The model under review builds one solid part; all positions refer to its coordinate system, in mm. A direction names the side the tool comes from. Give positions to 0.01 mm unless a question says otherwise; leave off trailing zeros. Loops run counter-clockwise (first coordinate to the right, second up) from the corner with the lowest first, then second, coordinate; pieces in that order, holes last. Notation, with made-up numbers: (20, 63) -> (65, 63) arc R23 ccw to (65, 93) -> close; hole circle Ø2 at (3, 42.5). An arc over 180 degrees is marked (long way). Write each question's results on one line, items separated by ' | '. Start each with the question number.
Q1. We need section B-B (y = 10.5). Write out the cut boundary in (x, z).
Q2. Machinability: for faces 5 (the face through (-33, 27, -40.018)), 6 (the face through (-65, 34, -17.018)), 7 (the face through (-107.678, 12, -33)), 8 (the face through (-24.8, 28.5, -30.7)), which of the approach directions +Z, -Z, +X, -X, +Y, -Y give a long, thin tool a straight path to every point of the face, cutting with its end or side? Answer none if there is none.
Q3. Wall thickness on L1, parallel to Z at x = -12.5, y = 3; L2, parallel to Y at x = -61, z = -35; L3, parallel to X at y = 5, z = -46: over which ranges is each line inside the solid? List them lowest first. Write a range as [from, to].
Q4. Mouldability with a two-part tool opening along Y and no side actions: class faces 1 (the face through (-75.451, 13.339, -45.483)), 2 (the face through (-102, 38, -15)), 3 (the face through (-108, 25, -48.018)), 4 (the face through (-66.044, 15.737, -15.483)) as released by +Y, released by -Y, zero draft, split by the parting line, or undercut.
Q5. We need section A-A (x = -50.5). Write out the cut boundary in (y, z).
Q6. We need section C-C (z = -30.5). Write out the cut boundary in (x, y), plus the area to 3 significant figures.
Q7. We need section D-D (y = 16.5). Write out the cut boundary in (x, z).
Q8. Insertion check: pin 1 Ø1.3 at (x, y) = (-101, 24) entering from -Z; pin 2 Ø12 at (x, z) = (-32, -16) entering from +Y; pin 3 Ø2 at (y, z) = (26.5, -35) entering from +X; pin 4 Ø1 at (x, z) = (-59.5, -11.5) entering from -Y. Each pin has a flat end and moves straight along its axis. Give the tip position at first contact, or say it passes through.
from build123d import *

# Parameters (mm, degrees)
BOSS_EXTRUDE3_DEPTH       = 30
SKETCH6_W                 = 25
SKETCH6_H                 = 23
CUT_EXTRUDE1_DEPTH        = 86
SKETCH7_W                 = 25
SKETCH7_H                 = 5
CUT_EXTRUDE2_DEPTH        = 7.5
SKETCH8_W                 = 25
SKETCH8_H                 = 2
CUT_EXTRUDE3_DEPTH        = 1
SKETCH9_R                 = 19
CUT_EXTRUDE4_DEPTH        = 5
BOSS_EXTRUDE4_DEPTH       = 30
SKETCH10_W                = 1.856561782
SKETCH10_H                = 30
BOSS_EXTRUDE5_DEPTH       = 3
BOSS_EXTRUDE6_DEPTH       = 30
SKETCH11_W                = 2.5
SKETCH11_H                = 23
CUT_EXTRUDE5_DEPTH        = 34.579503854
SKETCH12_W                = 29.135235428
SKETCH12_H                = 25
CUT_EXTRUDE6_DEPTH        = 3.5
SKETCH13_W                = 19.135235428
SKETCH13_H                = 5
CUT_EXTRUDE7_DEPTH        = 3.5
SKETCH14_W                = 29.135235428
SKETCH14_H                = 4
BOSS_EXTRUDE7_DEPTH       = 2
SKETCH16_W                = 29.135235428
SKETCH16_H                = 1.5
BOSS_EXTRUDE8_DEPTH       = 2
SKETCH17_W                = 2.551467674
SKETCH17_H                = 30
BOSS_EXTRUDE9_DEPTH       = 5
BOSS_EXTRUDE10_REACH      = 85.266
SKETCH18_W                = 29.135235428
SKETCH18_H                = 2.5
SKETCH19_W                = 2.48850009
SKETCH19_H                = 23
BOSS_EXTRUDE11_DEPTH      = 2
CUT_EXTRUDE8_START        = -2.4885
SKETCH20_W                = 2
SKETCH20_H                = 23
CUT_EXTRUDE8_DEPTH        = 21.736568
BOSS_EXTRUDE12_REACH      = 82.714
SKETCH21_W                = 2.023287715
SKETCH21_H                = 27.5
SKETCH22_W                = 35
SKETCH22_H                = 30
BOSS_EXTRUDE13_DEPTH      = 15.9
BOSS_EXTRUDE13_DEPTH_BACK = 7.5
SKETCH23_W                = 25
SKETCH23_H                = 23
CUT_EXTRUDE9_DEPTH        = 24.4
SKETCH24_W                = 25
SKETCH24_H                = 5
CUT_EXTRUDE10_DEPTH       = 2
SKETCH25_W                = 50
SKETCH25_H                = 29
CUT_EXTRUDE11_DEPTH       = 4
SKETCH26_W                = 3
SKETCH26_H                = 29
BOSS_EXTRUDE14_DEPTH      = 2.5
SKETCH27_W                = 5
SKETCH27_H                = 5
BOSS_EXTRUDE15_DEPTH      = 2.5
BOSS_EXTRUDE16_REACH      = 27
SKETCH28_W                = 4
SKETCH28_H                = 2.5
SKETCH29_W                = 13
SKETCH29_H                = 5
BOSS_EXTRUDE17_DEPTH      = 2.5
SKETCH30_W                = 10
SKETCH30_H                = 4
CUT_EXTRUDE12_DEPTH       = 14
CUT_EXTRUDE13_REACH       = 43.166
SKETCH31_W                = 10
SKETCH31_H                = 2
SKETCH32_W                = 2
SKETCH32_H                = 25
CUT_EXTRUDE14_DEPTH       = 27
SKETCH33_W                = 20.479278159
SKETCH33_H                = 4
BOSS_EXTRUDE18_DEPTH      = 8
SKETCH34_W                = 15.845031547
SKETCH34_H                = 4
BOSS_EXTRUDE19_DEPTH      = 8


with BuildPart() as part:
    # Sketch2 → Boss-Extrude3 (new body)
    with BuildSketch(Plane(origin=(0, 0, 0), x_dir=(1, 0, 0), z_dir=(0, 1, 0))):
        Polygon((-105.912162162, 13.018018018), (-20.912162162, 13.018018018), (-20.912162162, 48.018018018), (-75.912162162, 48.018018018), align=None)
    extrude(amount=BOSS_EXTRUDE3_DEPTH)

    # Sketch6 → Cut-Extrude1 (cut, through all)
    with BuildSketch(Plane(origin=(-20.912162162, 0, 0), x_dir=(0, 0, -1), z_dir=(1, 0, 0))):
        with Locations((30.518018018, 13.5)):
            Rectangle(SKETCH6_W, SKETCH6_H)
    extrude(amount=-CUT_EXTRUDE1_DEPTH, mode=Mode.SUBTRACT)

    # Sketch7 → Cut-Extrude2 (cut)
    with BuildSketch(Plane(origin=(-20.912162162, 0, 0), x_dir=(0, 0, -1), z_dir=(1, 0, 0))):
        with Locations((30.518018018, 27.5)):
            Rectangle(SKETCH7_W, SKETCH7_H)
    extrude(amount=-CUT_EXTRUDE2_DEPTH, mode=Mode.SUBTRACT)

    # Sketch8 → Cut-Extrude3 (cut)
    with BuildSketch(Plane(origin=(-20.912162162, 0, 0), x_dir=(0, 0, -1), z_dir=(1, 0, 0))):
        with Locations((30.518018018, 1)):
            Rectangle(SKETCH8_W, SKETCH8_H)
    extrude(amount=-CUT_EXTRUDE3_DEPTH, mode=Mode.SUBTRACT)

    # Sketch9 → Cut-Extrude4 (cut)
    with BuildSketch(Plane.XY.offset(-13.018018018)):
        with Locations((-84.912162162, 13.5)):
            Circle(SKETCH9_R)
    extrude(amount=-CUT_EXTRUDE4_DEPTH, mode=Mode.SUBTRACT)

    # Sketch3 → Boss-Extrude4 (add)
    with BuildSketch(Plane(origin=(0, 0, 0), x_dir=(1, 0, 0), z_dir=(0, 1, 0))):
        Polygon((-106.412808957, 7.383361614), (-110.17791555, 11.88278259), (-79.204856611, 48.018018018), (-75.912162162, 48.018018018), (-105.912162162, 13.018018018), (-103.345157358, 9.950366419), align=None)
    extrude(amount=BOSS_EXTRUDE4_DEPTH)

    # Sketch10 → Boss-Extrude5 (add)
    with BuildSketch(Plane.XY.offset(-13.018018018)):
        with Locations((-104.983881271, 15)):
            Rectangle(SKETCH10_W, SKETCH10_H)
    extrude(amount=BOSS_EXTRUDE5_DEPTH)

    # Sketch4 → Boss-Extrude6 (add)
    with BuildSketch(Plane(origin=(0, 0, 0), x_dir=(1, 0, 0), z_dir=(0, 1, 0))):
        Polygon((-110.17791555, 11.88278259), (-110.17791555, 48.018018018), (-104.17791555, 48.018018018), (-104.17791555, 18.88278259), align=None)
    extrude(amount=BOSS_EXTRUDE6_DEPTH)

    # Sketch11 → Cut-Extrude5 (cut, through all)
    with BuildSketch(Plane(origin=(-47.459390138, 0, -56.715466139), x_dir=(0.7669129, 0, -0.641751201), z_dir=(0.641751201, 0, 0.7669129))):
        with Locations((-74.121074711, 13.5)):
            Rectangle(SKETCH11_W, SKETCH11_H)
    extrude(amount=-CUT_EXTRUDE5_DEPTH, mode=Mode.SUBTRACT)

    # Sketch12 → Cut-Extrude6 (cut)
    with BuildSketch(Plane(origin=(-104.17791555, 0, 0), x_dir=(0, 0, -1), z_dir=(1, 0, 0))):
        with Locations((33.450400304, 15)):
            Rectangle(SKETCH12_W, SKETCH12_H)
    extrude(amount=-CUT_EXTRUDE6_DEPTH, mode=Mode.SUBTRACT)

    # Sketch13 → Cut-Extrude7 (cut, through all)
    with BuildSketch(Plane(origin=(-107.67791555, 0, 0), x_dir=(0, 0, -1), z_dir=(1, 0, 0))):
        with Locations((38.450400304, 15)):
            Rectangle(SKETCH13_W, SKETCH13_H)
    extrude(amount=-CUT_EXTRUDE7_DEPTH, mode=Mode.SUBTRACT)

    # Sketch14 → Boss-Extrude7 (add)
    with BuildSketch(Plane(origin=(-107.67791555, 0, 0), x_dir=(0, 0, -1), z_dir=(1, 0, 0))):
        with Locations((33.450400304, 25.5)):
            Rectangle(SKETCH14_W, SKETCH14_H)
    extrude(amount=BOSS_EXTRUDE7_DEPTH)

    # Sketch16 → Boss-Extrude8 (add)
    with BuildSketch(Plane(origin=(-107.67791555, 0, 0), x_dir=(0, 0, -1), z_dir=(1, 0, 0))):
        with Locations((33.450400304, 3.25)):
            Rectangle(SKETCH16_W, SKETCH16_H)
    extrude(amount=BOSS_EXTRUDE8_DEPTH)

    # Sketch17 → Boss-Extrude9 (add)
    with BuildSketch(Plane(origin=(0, 0, -18.88278259), x_dir=(-1, 0, 0), z_dir=(0, 0, -1))):
        with Locations((102.902181713, 15)):
            Rectangle(SKETCH17_W, SKETCH17_H)
    extrude(amount=BOSS_EXTRUDE9_DEPTH)

    # Boss-Extrude10: up to this face of the body (flat: up to its plane)
    boss_extrude10_end = Plane(part.part.faces().sort_by_distance((-90.415652244, 15, -34.938756447))[0])
    # Sketch18 → Boss-Extrude10 (add, up to the picked face)
    with BuildSketch(Plane(origin=(-104.17791555, 0, 0), x_dir=(0, 0, -1), z_dir=(1, 0, 0)), mode=Mode.PRIVATE) as boss_extrude10_sk1:
        with Locations((33.450400304, 1.25)):
            Rectangle(SKETCH18_W, SKETCH18_H)
    boss_extrude10_tool1 = split(extrude(boss_extrude10_sk1.sketch, amount=BOSS_EXTRUDE10_REACH, mode=Mode.PRIVATE), bisect_by=boss_extrude10_end, keep=Keep.BOTH, mode=Mode.PRIVATE)
    add(boss_extrude10_tool1.solids().sort_by_distance((-104.177916, 1.25, -33.4504))[0])

    # Sketch19 → Boss-Extrude11 (add)
    with BuildSketch(Plane(origin=(-67.487678855, 0, -57.846581876), x_dir=(0.650791373, 0, -0.759256602), z_dir=(0.759256602, 0, 0.650791373))):
        with Locations((-31.723015124, 13.5)):
            Rectangle(SKETCH19_W, SKETCH19_H)
    extrude(amount=BOSS_EXTRUDE11_DEPTH)

    # Sketch20 → Cut-Extrude8 (cut)
    with BuildSketch(Plane(origin=(-19.835317387, 0, 23.141203618), x_dir=(-0.759256602, 0, -0.650791373), z_dir=(0.650791373, 0, -0.759256602)).offset(CUT_EXTRUDE8_START)):
        with Locations((87.886522218, 13.5)):
            Rectangle(SKETCH20_W, SKETCH20_H)
    extrude(amount=CUT_EXTRUDE8_DEPTH, mode=Mode.SUBTRACT)

    # Boss-Extrude12: up to this face of the body (flat: up to its plane)
    boss_extrude12_end = Plane(part.part.faces().sort_by_distance((-90.415652244, 16.25, -34.938756447))[0])
    # Sketch21 → Boss-Extrude12 (add, up to the picked face)
    with BuildSketch(Plane(origin=(-101.626447876, 0, 0), x_dir=(0, 0, -1), z_dir=(1, 0, 0)), mode=Mode.PRIVATE) as boss_extrude12_sk1:
        with Locations((22.871138733, 16.25)):
            Rectangle(SKETCH21_W, SKETCH21_H)
    boss_extrude12_tool1 = split(extrude(boss_extrude12_sk1.sketch, amount=BOSS_EXTRUDE12_REACH, mode=Mode.PRIVATE), bisect_by=boss_extrude12_end, keep=Keep.BOTH, mode=Mode.PRIVATE)
    add(boss_extrude12_tool1.solids().sort_by_distance((-101.626448, 16.25, -22.871139))[0])

    # Sketch22 → Boss-Extrude13 (add, two sides)
    with BuildSketch(Plane(origin=(-20.912162162, 0, 0), x_dir=(0, 0, -1), z_dir=(1, 0, 0))) as boss_extrude13_sk:
        with Locations((30.518018018, 15)):
            Rectangle(SKETCH22_W, SKETCH22_H)
    extrude(amount=BOSS_EXTRUDE13_DEPTH)
    extrude(boss_extrude13_sk.sketch, amount=-BOSS_EXTRUDE13_DEPTH_BACK)

    # Sketch23 → Cut-Extrude9 (cut, through all)
    with BuildSketch(Plane.ZY.offset(28.412162162)):
        with Locations((-30.518018018, 13.5)):
            Rectangle(SKETCH23_W, SKETCH23_H)
    extrude(amount=-CUT_EXTRUDE9_DEPTH, mode=Mode.SUBTRACT)

    # Sketch24 → Cut-Extrude10 (cut)
    with BuildSketch(Plane(origin=(-5.012162162, 0, 0), x_dir=(0, 0, -1), z_dir=(1, 0, 0))):
        with Locations((30.518018018, 27.5)):
            Rectangle(SKETCH24_W, SKETCH24_H)
    extrude(amount=-CUT_EXTRUDE10_DEPTH, mode=Mode.SUBTRACT)

    # Sketch25 → Cut-Extrude11 (cut)
    with BuildSketch(Plane(origin=(0, 30, 0), x_dir=(1, 0, 0), z_dir=(0, 1, 0))):
        with Locations((-30.012162162, 30.518018018)):
            Rectangle(SKETCH25_W, SKETCH25_H)
    extrude(amount=-CUT_EXTRUDE11_DEPTH, mode=Mode.SUBTRACT)

    # Sketch26 → Boss-Extrude14 (add)
    with BuildSketch(Plane(origin=(0, 26, 0), x_dir=(1, 0, 0), z_dir=(0, 1, 0))):
        with Locations((-23.512162162, 30.518018018)):
            Rectangle(SKETCH26_W, SKETCH26_H)
    extrude(amount=BOSS_EXTRUDE14_DEPTH)

    # Sketch27 → Boss-Extrude15 (add)
    with BuildSketch(Plane(origin=(0, 26, 0), x_dir=(1, 0, 0), z_dir=(0, 1, 0))):
        with Locations((-32.512162162, 42.518018018)):
            Rectangle(SKETCH27_W, SKETCH27_H)
    extrude(amount=BOSS_EXTRUDE15_DEPTH)

    # Sketch28 → Boss-Extrude16 (add, up to next)
    with BuildSketch(Plane(origin=(-30.012162162, 0, 0), x_dir=(0, 0, -1), z_dir=(1, 0, 0)), mode=Mode.PRIVATE) as boss_extrude16_sk1:
        with Locations((43.018018018, 27.25)):
            Rectangle(SKETCH28_W, SKETCH28_H)
    boss_extrude16_tool1 = extrude(boss_extrude16_sk1.sketch, amount=BOSS_EXTRUDE16_REACH, mode=Mode.PRIVATE) - part.part
    add(boss_extrude16_tool1.solids().sort_by_distance((-30.012162, 27.25, -43.018018))[0])

    # Sketch29 → Boss-Extrude17 (add)
    with BuildSketch(Plane(origin=(0, 26, 0), x_dir=(1, 0, 0), z_dir=(0, 1, 0))):
        with Locations((-31.512162162, 18.518018018)):
            Rectangle(SKETCH29_W, SKETCH29_H)
    extrude(amount=BOSS_EXTRUDE17_DEPTH)

    # Sketch30 → Cut-Extrude12 (cut)
    with BuildSketch(Plane(origin=(-55.012162162, 0, 0), x_dir=(0, 0, -1), z_dir=(1, 0, 0))):
        with Locations((37.018018018, 28)):
            Rectangle(SKETCH30_W, SKETCH30_H)
    extrude(amount=-CUT_EXTRUDE12_DEPTH, mode=Mode.SUBTRACT)

    # Sketch31 → Cut-Extrude13 (cut, up to next)
    with BuildSketch(Plane(origin=(-69.012162162, 0, 0), x_dir=(0, 0, -1), z_dir=(1, 0, 0)), mode=Mode.PRIVATE) as cut_extrude13_sk1:
        with Locations((37.018018018, 29)):
            Rectangle(SKETCH31_W, SKETCH31_H)
    cut_extrude13_tool1 = extrude(cut_extrude13_sk1.sketch, amount=-CUT_EXTRUDE13_REACH, mode=Mode.PRIVATE) & part.part
    add(cut_extrude13_tool1.solids().sort_by_distance((-69.012162, 29, -37.018018))[0], mode=Mode.SUBTRACT)

    # Sketch32 → Cut-Extrude14 (cut, through all)
    with BuildSketch(Plane(origin=(0, 26, 0), x_dir=(1, 0, 0), z_dir=(0, 1, 0))):
        with Locations((-6.012162162, 30.518018018)):
            Rectangle(SKETCH32_W, SKETCH32_H)
    extrude(amount=-CUT_EXTRUDE14_DEPTH, mode=Mode.SUBTRACT)

    # Sketch33 → Boss-Extrude18 (add)
    with BuildSketch(Plane(origin=(0, 30, 0), x_dir=(1, 0, 0), z_dir=(0, 1, 0))):
        with Locations((-65.251801242, 15.018018018)):
            Rectangle(SKETCH33_W, SKETCH33_H)
    extrude(amount=BOSS_EXTRUDE18_DEPTH)

    # Sketch34 → Boss-Extrude19 (add)
    with BuildSketch(Plane(origin=(0, 30, 0), x_dir=(1, 0, 0), z_dir=(0, 1, 0))):
        with Locations((-102.255399777, 15.018018018)):
            Rectangle(SKETCH34_W, SKETCH34_H)
    extrude(amount=BOSS_EXTRUDE19_DEPTH)


solid = part.part
Output:
1) outline: (-110.18, -48.02) -> (-107.68, -48.02) -> (-107.68, -18.88) -> (-104.18, -18.88) -> (-104.18, -23.88) -> (-99.89, -23.88) -> (-79.2, -48.02) -> (-75.91, -48.02) -> (-103.67, -15.63) -> (-103.67, -13.02) -> (-104.06, -13.02) -> (-104.06, -10.8) -> (-110.18, -18.12) -> close; (-110.18, -14.22) -> (-105.26, -8.35) -> (-106.41, -7.38) -> (-110.18, -11.88) -> close; (-77.56, -43.02) -> (-73.28, -48.02) -> (-5.01, -48.02) -> (-5.01, -43.02) -> close; (-66.15, -18.02) -> (-5.01, -18.02) -> (-5.01, -13.02) -> (-66.15, -13.02) -> close
2) face 5: +Y | face 6: -Z, +X, -X, +Y | face 7: -Z | face 8: +X, +Y
3) L1: [-48.02, -43.02], [-18.02, -13.02] | L2: [0, 2], [25, 26] | L3: [-110.18, -107.68], [-80.93, -77.64], [-75.01, -5.01]
4) face 1: undercut | face 2: released by +Y | face 3: zero draft | face 4: undercut
5) outline: (0, -48.02) -> (30, -48.02) -> (30, -45.02) -> (26, -45.02) -> (26, -16.02) -> (30, -16.02) -> (30, -13.02) -> (0, -13.02) -> close; hole (2, -43.02) -> (25, -43.02) -> (25, -18.02) -> (2, -18.02) -> close
6) outline: (-110.18, 0) -> (-7.01, 0) -> (-7.01, 2) -> (-90.93, 2) -> (-90.93, 25) -> (-7.01, 25) -> (-7.01, 26) -> (-22.01, 26) -> (-22.01, 28.5) -> (-25.01, 28.5) -> (-25.01, 26) -> (-55.01, 26) -> (-55.01, 30) -> (-94.22, 30) -> (-94.22, 2.5) -> (-105.68, 2.5) -> (-105.68, 4) -> (-107.68, 4) -> (-107.68, 12.5) -> (-110.18, 12.5) -> close; (-110.18, 17.5) -> (-107.68, 17.5) -> (-107.68, 23.5) -> (-105.68, 23.5) -> (-105.68, 27.5) -> (-104.18, 27.5) -> (-104.18, 30) -> (-110.18, 30) -> close | area: 618 mm2
7) outline: (-110.18, -28.88) -> (-107.68, -28.88) -> (-107.68, -18.88) -> (-104.18, -18.88) -> (-104.18, -23.88) -> (-99.89, -23.88) -> (-79.2, -48.02) -> (-75.91, -48.02) -> (-103.67, -15.63) -> (-103.67, -13.02) -> (-104.06, -13.02) -> (-104.06, -10.8) -> (-110.18, -18.12) -> close; (-110.18, -14.22) -> (-105.26, -8.35) -> (-106.41, -7.38) -> (-110.18, -11.88) -> close; (-77.56, -43.02) -> (-73.28, -48.02) -> (-5.01, -48.02) -> (-5.01, -43.02) -> close; (-66.15, -18.02) -> (-5.01, -18.02) -> (-5.01, -13.02) -> (-66.15, -13.02) -> close
8) pin 1: z = -23.88 | pin 2: y = 30 | pin 3: x = -7.01 | pin 4: through
